from build123d import *

# Parameters (mm, degrees)
IZIM1_W                     = 220
IZIM1_H                     = 140
Y_KSEKLIK_EKSTR_ZYON1_DEPTH = 3
IZIM2_R                     = 2
KES_EKSTR_ZYON1_DEPTH       = 3


with BuildPart() as part:
    # Çizim1 → Yükseklik-Ekstrüzyon1 (new body)
    with BuildSketch(Plane.XY):
        with Locations((110, 70)):
            Rectangle(IZIM1_W, IZIM1_H)
    extrude(amount=Y_KSEKLIK_EKSTR_ZYON1_DEPTH)

    # Çizim2 → Kes-Ekstrüzyon1 (cut)
    with BuildSketch(Plane.XY.offset(3)):
        with Locations((15, 125)):
            Circle(IZIM2_R)
        with Locations((205, 125)):
            Circle(IZIM2_R)
        with Locations((110, 125)):
            Circle(IZIM2_R)
        with Locations(Location((205, 15, 0), (0, 0, 180))):
            Circle(IZIM2_R)
        with Locations(Location((110, 15, 0), (0, 0, 180))):
            Circle(IZIM2_R)
        with Locations(Location((15, 15, 0), (0, 0, 180))):
            Circle(IZIM2_R)
    extrude(amount=-KES_EKSTR_ZYON1_DEPTH, mode=Mode.SUBTRACT)


solid = part.part
Geometry check sheet. Reference: the model listing, model coordinates, mm. Give positions to 0.01 mm unless a question says otherwise; leave off trailing zeros.
1) Draft check along Y on faces 1 (the flat face through (108, 71, 3)), 2 (the cylindrical face through (207, 15, 2)). Enter one of: released by +Y, released by -Y, zero draft, split by the parting line, or undercut.
Results are:
face 1: zero draft
face 2: undercut
2) Material ranges on probe 1 along Y at (x, z) = (205, 1.5); probe 2 along X at (y, z) = (15, 0.7); probe 3 along X at (y, z) = (16.5, 2.4), recorded low to high.
Results are:
probe 1: y = 0 to 13, 17 to 123, 127 to 140
probe 2: x = 0 to 13, 17 to 108, 112 to 203, 207 to 220
probe 3: x = 0 to 13.68, 16.32 to 108.68, 111.32 to 203.68, 206.32 to 220
3) Gauge pin test, flat end, axial feed: pin 1 (3.5 mm diameter, centred on x = 110, y = 125, fed in from -Z). Record the tip position at first contact, or that the pin passes through.
Results are:
pin 1: passes through
